```python
from build123d import *

# Parameters (mm, degrees)
SKETCH218_AS_DRAWN_R                    = 1.85
EXTRUDE136003_DEPTH                     = 20
EXTRUDE136003_ONTO_SKETCH218_ROLL_ANGLE = 90
EXTRUDE136010_DEPTH                     = 50
SKETCH221_AS_DRAWN_R                    = 2.75
EXTRUDE136006_DEPTH                     = 9
EXTRUDE136006_ONTO_SKETCH221_ROLL_ANGLE = 90
SKETCH220_AS_DRAWN_R                    = 1.85
EXTRUDE136005_DEPTH                     = 20
EXTRUDE136005_ONTO_SKETCH220_ROLL_ANGLE = 90
EXTRUDE136004_DEPTH                     = 38
EXTRUDE136011_DEPTH                     = 50
SKETCH224_AS_DRAWN_R                    = 2.75
EXTRUDE136009_DEPTH                     = 9
EXTRUDE136009_ONTO_SKETCH224_ROLL_ANGLE = 90
SKETCH223_AS_DRAWN_R                    = 1.85
EXTRUDE136008_DEPTH                     = 20
EXTRUDE136008_ONTO_SKETCH223_ROLL_ANGLE = 90
EXTRUDE136007_DEPTH                     = 24
EXTRUDE136012_DEPTH                     = 14
SKETCH227_W                             = 9.75
SKETCH227_H                             = 16.75
EXTRUDE136013_DEPTH                     = 9
EXTRUDE136014_DEPTH                     = 7
EXTRUDE136002_DEPTH                     = 128


with BuildPart() as extrude136003:
    # Sketch218 as drawn → Extrude136003 (new)
    with BuildSketch(Plane.XY):
        with Locations((0, -9)):
            Circle(SKETCH218_AS_DRAWN_R)
        Polygon((3.5, 19.187822), (7, 25.25), (3.5, 31.312178), (-3.5, 31.312178), (-7, 25.25), (-3.5, 19.187822), align=None)
        Polygon((3.5, 35.187822), (7, 41.25), (3.5, 47.312178), (-3.5, 47.312178), (-7, 41.25), (-3.5, 35.187822), align=None)
        Polygon((3.5, 51.187822), (7, 57.25), (3.5, 63.312178), (-3.5, 63.312178), (-7, 57.25), (-3.5, 51.187822), align=None)
        Polygon((3.5, 67.187822), (7, 73.25), (3.5, 79.312178), (-3.5, 79.312178), (-7, 73.25), (-3.5, 67.187822), align=None)
        Polygon((3.5, 83.187822), (7, 89.25), (3.5, 95.312178), (-3.5, 95.312178), (-7, 89.25), (-3.5, 83.187822), align=None)
        Polygon((3.5, 99.187822), (7, 105.25), (3.5, 111.312178), (-3.5, 111.312178), (-7, 105.25), (-3.5, 99.187822), align=None)
        Polygon((3.5, 115.187822), (7, 121.25), (3.5, 127.312178), (-3.5, 127.312178), (-7, 121.25), (-3.5, 115.187822), align=None)
        Polygon((3.5, 131.187822), (7, 137.25), (3.5, 143.312178), (-3.5, 143.312178), (-7, 137.25), (-3.5, 131.187822), align=None)
        with BuildLine():
            Line((5, -8.999981), (5, -15.999981))
            Line((5, -15.999981), (-5, -15.999981))
            Line((-5, -15.999981), (-5, -8.999981))
            ThreePointArc((-5, -8.999981), (0, -14), (5, -8.999981))
        make_face()
    extrude(amount=-EXTRUDE136003_DEPTH)


with BuildPart() as extrude136003_1:
    # Extrude136003 onto Sketch218 roll: moved
    add(extrude136003.part.rotate(Axis((0, 0, 0), (1, 0, 0)), EXTRUDE136003_ONTO_SKETCH218_ROLL_ANGLE))


with BuildPart() as extrude136003_2:
    # Extrude136003 onto Sketch218 placement: moved
    add(extrude136003_1.part)


with BuildPart() as extrude136010:
    # Sketch225 → Extrude136010 (new body)
    with BuildSketch(Plane.YZ):
        Polygon((0, -9.814955), (17, 0), (17, -9.814955), align=None)
        Polygon((17, 29), (0, 19.185045), (0, 29), align=None)
    extrude(amount=EXTRUDE136010_DEPTH)


with BuildPart() as extrude136010_1:
    # Extrude136010 placement: moved
    add(extrude136010.part.moved(Location((-25, 0, 0))))


with BuildPart() as extrude136006:
    # Sketch221 as drawn → Extrude136006 (new)
    with BuildSketch(Plane.XY):
        with Locations((-16, 0)):
            Circle(SKETCH221_AS_DRAWN_R)
        with Locations((16, 0)):
            Circle(SKETCH221_AS_DRAWN_R)
    extrude(amount=-EXTRUDE136006_DEPTH)


with BuildPart() as extrude136006_1:
    # Extrude136006 onto Sketch221 roll: moved
    add(extrude136006.part.rotate(Axis((0, 0, 0), (1, 0, 0)), EXTRUDE136006_ONTO_SKETCH221_ROLL_ANGLE))


with BuildPart() as extrude136006_2:
    # Extrude136006 onto Sketch221 placement: moved
    add(extrude136006_1.part)


with BuildPart() as fusion034004041035:
    # Sketch220 as drawn → Extrude136005 (new)
    with BuildSketch(Plane.XY):
        with Locations((-16, 0)):
            Circle(SKETCH220_AS_DRAWN_R)
        with Locations((16, 0)):
            Circle(SKETCH220_AS_DRAWN_R)
    extrude(amount=-EXTRUDE136005_DEPTH)


with BuildPart() as fusion034004041035_1:
    # Extrude136005 onto Sketch220 roll: moved
    add(fusion034004041035.part.rotate(Axis((0, 0, 0), (1, 0, 0)), EXTRUDE136005_ONTO_SKETCH220_ROLL_ANGLE))


with BuildPart() as fusion034004041035_2:
    # Extrude136005 onto Sketch220 placement: moved
    add(fusion034004041035_1.part)

    # Fusion034004041033: union Extrude136006
    add(extrude136006_2.part)


with BuildPart() as fusion034004041035_3:
    # Fusion034004041033 placement: moved
    add(fusion034004041035_2.part.moved(Location((0, 0, 13))))

    # Fusion034004041035: union Extrude136010
    add(extrude136010_1.part)


with BuildPart() as cut009010006006004:
    # Sketch219 → Extrude136004 (new body)
    with BuildSketch(Plane.XY):
        with BuildLine():
            Line((-11, 0), (11, 0))
            Line((20.5, 11.321659), (11, 0))
            Line((20.5, 11.321659), (20.5, 16.890918))
            Line((20.5, 16.890918), (12.499524, 16.890918))
            ThreePointArc((-12.499524, 16.890918), (0, 4.5), (12.499524, 16.890918))
            Line((-20.5, 16.890918), (-12.499524, 16.890918))
            Line((-20.5, 11.321659), (-20.5, 16.890918))
            Line((-20.5, 11.321659), (-11, 0))
        make_face()
    extrude(amount=EXTRUDE136004_DEPTH)


with BuildPart() as cut009010006006004_1:
    # Extrude136004 placement: moved
    add(cut009010006006004.part.moved(Location((0, 0, -9))))

    # Cut009010006006004: cut Fusion034004041035
    add(fusion034004041035_3.part, mode=Mode.SUBTRACT)


with BuildPart() as cut009010006006004_2:
    # Cut009010006006004 placement: moved
    add(cut009010006006004_1.part.moved(Location((0, 0, 141))))


with BuildPart() as extrude136011:
    # Sketch226 → Extrude136011 (new body)
    with BuildSketch(Plane.YZ):
        Polygon((0, 24), (17, 24), (17, 14.185045), align=None)
    extrude(amount=EXTRUDE136011_DEPTH)


with BuildPart() as extrude136011_1:
    # Extrude136011 placement: moved
    add(extrude136011.part.moved(Location((-25, 0, 0))))


with BuildPart() as extrude136009:
    # Sketch224 as drawn → Extrude136009 (new)
    with BuildSketch(Plane.XY):
        with Locations((-16, 0)):
            Circle(SKETCH224_AS_DRAWN_R)
        with Locations((16, 0)):
            Circle(SKETCH224_AS_DRAWN_R)
    extrude(amount=-EXTRUDE136009_DEPTH)


with BuildPart() as extrude136009_1:
    # Extrude136009 onto Sketch224 roll: moved
    add(extrude136009.part.rotate(Axis((0, 0, 0), (1, 0, 0)), EXTRUDE136009_ONTO_SKETCH224_ROLL_ANGLE))


with BuildPart() as extrude136009_2:
    # Extrude136009 onto Sketch224 placement: moved
    add(extrude136009_1.part)


with BuildPart() as fusion034004041034:
    # Sketch223 as drawn → Extrude136008 (new)
    with BuildSketch(Plane.XY):
        with Locations((-16, 0)):
            Circle(SKETCH223_AS_DRAWN_R)
        with Locations((16, 0)):
            Circle(SKETCH223_AS_DRAWN_R)
    extrude(amount=-EXTRUDE136008_DEPTH)


with BuildPart() as fusion034004041034_1:
    # Extrude136008 onto Sketch223 roll: moved
    add(fusion034004041034.part.rotate(Axis((0, 0, 0), (1, 0, 0)), EXTRUDE136008_ONTO_SKETCH223_ROLL_ANGLE))


with BuildPart() as fusion034004041034_2:
    # Extrude136008 onto Sketch223 placement: moved
    add(fusion034004041034_1.part)

    # Fusion034004041034: union Extrude136009
    add(extrude136009_2.part)


with BuildPart() as fusion034004041034_3:
    # Fusion034004041034 placement: moved
    add(fusion034004041034_2.part.moved(Location((0, 0, 9))))


with BuildPart() as cut009010006006005:
    # Sketch222 → Extrude136007 (new body)
    with BuildSketch(Plane.XY):
        with BuildLine():
            Line((-11, 0), (11, 0))
            Line((20.5, 11.321659), (11, 0))
            Line((20.5, 11.321659), (20.5, 16.890918))
            Line((20.5, 16.890918), (12.499524, 16.890918))
            ThreePointArc((-12.499524, 16.890918), (0, 4.5), (12.499524, 16.890918))
            Line((-20.5, 16.890918), (-12.499524, 16.890918))
            Line((-20.5, 11.321659), (-20.5, 16.890918))
            Line((-20.5, 11.321659), (-11, 0))
        make_face()
    extrude(amount=EXTRUDE136007_DEPTH)

    # Cut009010006006003: cut Fusion034004041034
    add(fusion034004041034_3.part, mode=Mode.SUBTRACT)

    # Cut009010006006005: cut Extrude136011
    add(extrude136011_1.part, mode=Mode.SUBTRACT)


with BuildPart() as extrude136012:
    # Sketch199 → Extrude136012 (new body)
    with BuildSketch(Plane.XY):
        with BuildLine():
            Line((-4.875, 0), (4.875, 0))
            Line((4.875, 5.489814), (4.875, 0))
            ThreePointArc((-4.875, 5.489814), (0, 4.5), (4.875, 5.489814))
            Line((-4.875, 5.489814), (-4.875, 0))
        make_face()
    extrude(amount=-EXTRUDE136012_DEPTH)


with BuildPart() as extrude136013:
    # Sketch227 → Extrude136013 (new body)
    with BuildSketch(Plane.XY):
        with Locations((0, 8.375)):
            Rectangle(SKETCH227_W, SKETCH227_H)
    extrude(amount=-EXTRUDE136013_DEPTH)


with BuildPart() as extrude136013_1:
    # Extrude136013 placement: moved
    add(extrude136013.part.moved(Location((0, 0, -5))))


with BuildPart() as extrude136014:
    # Sketch228 → Extrude136014 (new body)
    with BuildSketch(Plane.XY):
        Polygon((0, 5), (0, 0), (-20.5, 0), (-22.665064, 3.75), (-22.665064, 11.75), (-20.5, 15.5), (-18, 15.5), (-18, 13), (-18.665064, 11.848076), (-18.665064, 6.151924), (-18, 5), align=None)
    extrude(amount=EXTRUDE136014_DEPTH)


with BuildPart() as extrude136014_1:
    # Extrude136014 placement: moved
    add(extrude136014.part.moved(Location((0, 0, 101))))


with BuildPart() as cut009010006006006:
    # Sketch217 → Extrude136002 (new body)
    with BuildSketch(Plane.XY):
        with BuildLine():
            Line((-11, 0), (11, 0))
            Line((11, 0), (12.678199, 2))
            Line((12.678199, 2), (7.609518, 7.083083))
            ThreePointArc((-7.609518, 7.083083), (0, 4.5), (7.609518, 7.083083))
            Line((-12.678199, 2), (-7.609518, 7.083083))
            Line((-11, 0), (-12.678199, 2))
        make_face()
    extrude(amount=EXTRUDE136002_DEPTH)


with BuildPart() as cut009010006006006_1:
    # Extrude136002 placement: moved
    add(cut009010006006006.part.moved(Location((0, 0, 17))))

    # Fusion034004041036: union Cut009010006006004, Cut009010006006005, Extrude136012, Extrude136013, Extrude136014
    add(cut009010006006004_2.part)
    add(cut009010006006005.part)
    add(extrude136012.part)
    add(extrude136013_1.part)
    add(extrude136014_1.part)

    # Cut009010006006006: cut Extrude136003
    add(extrude136003_2.part, mode=Mode.SUBTRACT)


solid = cut009010006006006_1.part
```
Input: part model. Units: mm. Frame: model coordinates. A direction names the side the tool comes from. Round coordinates to 2 decimals unless told otherwise and drop trailing zeros. Loops run counter-clockwise (first coordinate to the right, second up) from the corner with the lowest first, then second, coordinate; pieces in that order, holes last. Notation, with made-up numbers: (35.5, 70.5) - (88.5, 70.5) arc R5 cw to (88.5, 76.5) - close; hole circle Ø2 at (44, 39.5). An arc over 180 degrees is marked (long way). One line per item, written item: value. Start each with the question number.
(1) Contact query for flat-ended pins moving along their axis: P1, Ø4, axis at x = 1.5, y = 3.5, coming from the +Z side; P2, Ø5, axis at x = 11.5, y = 8.5, coming from the -Z side; P3, Ø0.8, axis at y = 14.5, z = 106, coming from the +X side; P4, Ø3.5, axis at x = -16, z = 154, coming from the +Y side. Output: stop coordinate, or through.
(2) Section C-C, the plane x = -16. Return loops of the section in (y, z), plus the area to 3 significant figures.
(3) Draft query along Z for faces 4 (the flat face through (13, 9, 0)), 5 (the flat face through (0, 2, 127.312)), 6 (the flat face through (18, 16.891, 155)). Return one class per face: +Z half, -Z half, draft (parallel to the pull), parting line (faces both ways), or undercut.
(4) Access query for faces 1 (the cylindrical face through (13.252, 6.406, 9.106)), 2 (the flat face through (-5.275, 2.537, 70.261)), 3 (the flat face through (-14.145, 10.996, 137.533)). Directions: +Z, -Z, +X, -X, +Y, -Y. A direction counts if a zero-diameter tool reaches every point of the face in a straight line with its end or side. Return the directions, or none.
(5) Section D-D, the plane z = 61.5. Return loops of the section in (x, y), plus the area to 3 significant figures.
(6) Section B-B, the plane x = 16. Return loops of the section in (y, z), plus the area to 3 significant figures.
(7) Ray query, line 1 (X direction, y = 14, z = 154); line 2 (Z direction, x = -16, y = 15); line 3 (Z direction, x = 16, y = 14.5). Return the intervals inside material, ascending. Write a range as [from, to].
(8) Section A-A, the plane z = 27.5. Return loops of the section in (x, y), plus the area to 3 significant figures.
Results below:
1. P1: z = 162.99
1. P2: z = 0
1. P3: x = -18
1. P4: through
2. outline: (0, 101) - (5, 101) - (5, 108) - (0, 108) - close; (5.96, 0) - (16.89, 0) - (16.89, 7.15) - (9, 7.15) - (9, 6.25) - (5.96, 6.25) - close; (5.96, 11.75) - (9, 11.75) - (9, 10.85) - (16.89, 10.85) - (16.89, 14.25) - (5.96, 20.56) - close; (5.96, 134.63) - (16.89, 140.94) - (16.89, 152.15) - (9, 152.15) - (9, 151.25) - (5.96, 151.25) - close; (5.96, 156.75) - (9, 156.75) - (9, 155.85) - (16.89, 155.85) - (16.89, 169.94) - (5.96, 163.63) - close
2. area: 450 mm^2
3. face 4: -Z half
3. face 5: undercut
3. face 6: draft
4. face 1: -Y
4. face 2: +Y, -Y
4. face 3: -X, +Y
5. outline: (-12.68, 2) - (-11, 0) - (-4.55, 0) - (-4.55, 5.36) arc R12.5 cw to (-7.61, 7.08) - close; (4.55, 0) - (11, 0) - (12.68, 2) - (7.61, 7.08) arc R12.5 cw to (4.55, 5.36) - close
5. area: 80.2 mm^2
6. outline: (5.96, 0) - (16.89, 0) - (16.89, 7.15) - (9, 7.15) - (9, 6.25) - (5.96, 6.25) - close; (5.96, 11.75) - (9, 11.75) - (9, 10.85) - (16.89, 10.85) - (16.89, 14.25) - (5.96, 20.56) - close; (5.96, 134.63) - (16.89, 140.94) - (16.89, 152.15) - (9, 152.15) - (9, 151.25) - (5.96, 151.25) - close; (5.96, 156.75) - (9, 156.75) - (9, 155.85) - (16.89, 155.85) - (16.89, 169.94) - (5.96, 163.63) - close
6. area: 415 mm^2
7. line 1: [-20.5, -17.85], [-14.15, -12.13], [12.13, 14.15], [17.85, 20.5]
7. line 2: [0, 7.15], [10.85, 15.34], [139.85, 152.15], [155.85, 168.85]
7. line 3: [0, 7.15], [10.85, 15.63], [139.56, 152.15], [155.85, 168.56]
8. outline: (-12.68, 2) - (-11, 0) - (-5.7, 0) - (-5.7, 5.88) arc R12.5 cw to (-7.61, 7.08) - close; (5.7, 0) - (11, 0) - (12.68, 2) - (7.61, 7.08) arc R12.5 cw to (5.7, 5.88) - close
8. area: 67.3 mm^2
